from build123d import *

# Parameters (mm, degrees)
F1_DEPTH = 12.7
F2_R     = 12.7
F3_DEPTH = 19.05
F4_W     = 12.7
F4_H     = 76.2
F4_R     = 6.35
F4_R_2   = 1.5875
F4_R_3   = 19.05
F5_DEPTH = 19.05
F6_DEPTH = 12.7
F7_R     = 1.5875
F8_DEPTH = 3.175


with BuildPart() as f1:
    # F0 (on Top) → F1 (new body)
    with BuildSketch(Plane.XY):
        Polygon((304.157444, 1142.615758), (-153.042556, 1142.615758), (-153.042556, 736.215758), (-229.242556, 736.215758), (-229.242556, -838.584242), (-63.805879, -838.584242), (380.357444, -838.584242), (380.357444, 736.215758), (304.157444, 736.215758), align=None)
    extrude(amount=F1_DEPTH)

    # F2 (on face) → F3 (cut)
    with BuildSketch(Plane.XY.offset(12.7)):
        Polygon((177.157444, -533.784242), (126.357444, -533.784242), (24.757444, -533.784242), (24.757444, -813.184242), (126.357444, -813.184242), (177.157444, -813.184242), align=None)
        with Locations((75.557444, 1091.815758)):
            Circle(F2_R)
    extrude(amount=-F3_DEPTH, mode=Mode.SUBTRACT)

    # F4 (on face) → F5 (cut)
    with BuildSketch(Plane.XY.offset(12.7)):
        with Locations((-153.042556, -667.134242)):
            Rectangle(F4_W, F4_H)
        with Locations((-153.042556, -514.734242)):
            Rectangle(F4_W, F4_H)
        with Locations((-153.042556, -362.334242)):
            Rectangle(F4_W, F4_H)
        with Locations((304.157444, -514.734242)):
            Rectangle(F4_W, F4_H)
        with Locations((304.157444, -667.134242)):
            Rectangle(F4_W, F4_H)
        with Locations((304.157444, -362.334242)):
            Rectangle(F4_W, F4_H)
        with Locations((227.957444, 761.615758)):
            Circle(F4_R)
        with Locations((-76.842556, 761.615758)):
            Circle(F4_R)
        with Locations((75.557444, 736.215758)):
            Circle(F4_R_2)
        with Locations((75.557444, 482.215758)):
            Circle(F4_R_3)
        with Locations((-51.442556, 660.015758)):
            Circle(F4_R)
    extrude(amount=-F5_DEPTH, mode=Mode.SUBTRACT)

    # F4 (on face) → F6 (cut)
    with BuildSketch(Plane.XY.offset(12.7)):
        with Locations((-153.042556, -667.134242)):
            Rectangle(F4_W, F4_H)
        with Locations((-153.042556, -514.734242)):
            Rectangle(F4_W, F4_H)
        with Locations((-153.042556, -362.334242)):
            Rectangle(F4_W, F4_H)
        with Locations((304.157444, -514.734242)):
            Rectangle(F4_W, F4_H)
        with Locations((304.157444, -667.134242)):
            Rectangle(F4_W, F4_H)
        with Locations((304.157444, -362.334242)):
            Rectangle(F4_W, F4_H)
        with Locations((227.957444, 761.615758)):
            Circle(F4_R)
        with Locations((-76.842556, 761.615758)):
            Circle(F4_R)
        with Locations((75.557444, 736.215758)):
            Circle(F4_R_2)
        with Locations((75.557444, 482.215758)):
            Circle(F4_R_3)
        with Locations((-51.442556, 660.015758)):
            Circle(F4_R)
    extrude(amount=-F6_DEPTH, mode=Mode.SUBTRACT)

    # F7 (on face) → F8 (join)
    with BuildSketch(Plane.XY.offset(12.7)):
        with Locations((75.557444, 736.215758)):
            Circle(F7_R)
    extrude(amount=-F8_DEPTH)


solid = f1.part
Could you check a few things on this model? Use its own coordinates, in mm. Give positions to 0.01 mm unless a question says otherwise; leave off trailing zeros. Order: outer loops, then holes, each group sorted by start corner. A loop starts at its lowest first (then second) coordinate and runs counter-clockwise, first axis right, second up. Notation, with made-up numbers: (26, 62.5) - (31, 62.5) arc R19 cw to (31, 84.5) - close; hole circle Ø10 at (-27, -24.75). An arc over 180 degrees is marked (long way). One line per question, with ' | ' between items. Start each with the question number.
Item 1: I want a section at D-D on z = 4. Give the number of separate pieces and of enclosed holes in the cut face, then the cut area to 3 significant figures.
Item 2: I'm going to push flat-ended pins straight in: pin 1 Ø4 at (x, z) = (307, 6) entering from +Y; pin 2 Ø15 at (x, y) = (75.56, 1091.82) entering from +Z. Where does each tip first touch, or does it pass through?
Item 3: I need wall thicknesses on probe 1 along Y at (x, z) = (-147, 4.25); probe 2 along Y at (x, z) = (136, 5.75); probe 3 along X at (y, z) = (842.5, 3.25). Which ranges of each line are inside material? Lowest first, please. Write a range as [from, to].
Item 4: I want a section at B-B on x = 142. Write out the boundary of the cut face in (y, z).
Item 5: Thinking about a two-plate mould opening in Y: for faces 1 (the flat face through (71, 166, 12.7)), 2 (the cylindrical face through (71.43, 463.62, 6.44)), which applies, pulls with the +Y half, pulls with the -Y half, needs draft (parallel to the pull), parting line crosses it, or undercut?
Item 6: I want a section at C-C on y = 960. Write out the boundary of the cut face in (x, z).
Item 7: I want a section at A-A on y = -581. Write out the boundary of the cut face in (x, z), then the cut area to 3 significant figures.
Verdict:
1) separate pieces: 1 | enclosed holes: 13 | area: 1,100,000 mm^2
2) pin 1: y = 736.22 | pin 2: through
3) probe 1: [-838.58, -705.23], [-629.03, -552.83], [-476.63, -400.43], [-324.23, 1142.62] | probe 2: [-838.58, -813.18], [-533.78, 1142.62] | probe 3: [-153.04, 304.16]
4) outline: (-838.58, 0) - (-813.18, 0) - (-813.18, 12.7) - (-838.58, 12.7) - close; (-533.78, 0) - (1142.62, 0) - (1142.62, 12.7) - (-533.78, 12.7) - close
5) face 1: needs draft | face 2: undercut
6) outline: (-153.04, 0) - (304.16, 0) - (304.16, 12.7) - (-153.04, 12.7) - close
7) outline: (-229.24, 0) - (24.76, 0) - (24.76, 12.7) - (-229.24, 12.7) - close; (177.16, 0) - (380.36, 0) - (380.36, 12.7) - (177.16, 12.7) - close | area: 5,810 mm^2
